Design review of the part built by this model. Coordinates are the model's own, in mm. A direction names the side the tool comes from. Coordinates: 2 decimals unless noted, no trailing zeros. Loops run counter-clockwise (first coordinate to the right, second up) from the corner with the lowest first, then second, coordinate; pieces in that order, holes last. Notation, with made-up numbers: (86, 33.5) -> (132, 33.5) arc R17 ccw to (132, 52.5) -> close; hole circle Ø3 at (-21, 51.25). An arc over 180 degrees is marked (long way). Use CSV: the item, a comma, the result in double quotes.
Autodesk Inventor part; units mm, degrees
ref_plane "YZ Plane" through (0, 0, 0) normal (1, 0, 0) x (0, 1, 0)
ref_plane "XZ Plane" through (0, 0, 0) normal (0, 1, 0) x (-1, 0, 0)
ref_plane "XY Plane" through (0, 0, 0) normal (0, 0, 1) x (1, 0, 0)
sketch "Sketch1" plane through (0, 0, 0) normal (0, 0, 1) x (1, 0, 0)
  circle A0 centre (482.6, 12.7) radius 3.302
  circle A1 centre (508, 241.3) radius 3.302
  circle A2 centre (482.6, 241.3) radius 3.302
  circle A3 centre (355.6, 241.3) radius 3.302
  circle A4 centre (330.2, 241.3) radius 3.302
  circle A5 centre (127, 63.5) radius 3.175
  circle A6 centre (127, 241.3) radius 3.175
  line L0 (427.3692, 9.8745) -> (431.8594, 5.3844)
  line L1 (431.8594, 5.3844) -> (485.7409, 59.2659)
  line L2 (485.7409, 59.2659) -> (481.2508, 63.7561)
  circle A7 centre (330.2, 63.5) radius 3.302
  circle A8 centre (254, 241.3) radius 3.302
  circle A9 centre (279.4, 63.5) radius 3.302
  circle A10 centre (355.6, 63.5) radius 3.302
  circle A11 centre (508, 63.5) radius 3.302
  circle A12 centre (355.6, 12.7) radius 3.302
  circle A13 centre (508, 12.7) radius 3.302
  line L3 (0, 254) -> (76.2, 254)
  line L4 (76.2, 254) -> (76.2, 260.35)
  line L5 (76.2, 260.35) -> (152.4, 260.35)
  line L6 (152.4, 260.35) -> (152.4, 254)
  line L7 (152.4, 254) -> (228.6, 254)
  line L8 (228.6, 254) -> (228.6, 260.35)
  line L9 (228.6, 260.35) -> (520.7, 260.35)
  line L10 (520.7, 260.35) -> (520.7, 0)
  line L11 (520.7, 0) -> (342.9, 0)
  line L12 (228.6, 44.45) -> (228.6, 50.8)
  line L13 (228.6, 50.8) -> (152.4, 50.8)
  line L14 (152.4, 50.8) -> (152.4, 44.45)
  line L15 (152.4, 44.45) -> (76.2, 44.45)
  line L16 (76.2, 44.45) -> (76.2, 50.8)
  line L17 (76.2, 50.8) -> (0, 50.8)
  line L18 (0, 50.8) -> (0, 254)
  line L19 (490.8349, 111.3178) -> (383.0718, 219.0809)
  line L20 (383.0718, 219.0809) -> (387.562, 223.571)
  line L21 (387.562, 223.571) -> (495.3, 115.7829)
  line L22 (495.3, 115.7829) -> (490.8349, 111.3178)
  line L23 (427.3692, 9.8745) -> (481.2508, 63.7561)
  circle A14 centre (279.4, 241.3) radius 3.302
  circle A15 centre (381, 241.3) radius 3.302
  circle A16 centre (254, 63.5) radius 3.302
  circle A17 centre (304.8, 241.3) radius 3.302
  circle A18 centre (304.8, 63.5) radius 3.302
  line L24 (266.7, 0) -> (342.9, 0)
  line L25 (266.7, 0) -> (266.7, 44.45)
  line L26 (228.6, 44.45) -> (266.7, 44.45)
  circle A19 centre (279.4, 12.7) radius 3.302
  point P0 (0, 0)
extrude "Extrusion2" add sketch "Sketch1" along normal blind 6.35
properties part number "vrRig_v8_side"
Item 1: To check wall thickness, follow line 1 along Y through (x, z) = (127, 2.75) (3 decimals); line 2 along Y through (x, z) = (304.8, 4); line 3 along Y through (x, z) = (508, 2.5). State the ranges of each line that lie inside material, in increasing order.
Checked values:
line 1,"44.45 to 60.325, 66.675 to 238.125, 244.475 to 260.35"
line 2,"0 to 60.2, 66.8 to 238, 244.6 to 260.35"
line 3,"0 to 9.4, 16 to 60.2, 66.8 to 238, 244.6 to 260.35"
Item 2: Add section B-B (x = 408). Give the boundary of the cut face in (y, z).
Checked values:
outline,"(0, 0) -> (194.15, 0) -> (194.15, 6.35) -> (0, 6.35) -> close; (203.12, 0) -> (260.35, 0) -> (260.35, 6.35) -> (203.12, 6.35) -> close"
Item 3: Add section C-C (z = 5). State how many separate pieces and enclosed holes the cut face has, then the cut area to 3 significant figures.
Checked values:
separate pieces,"1"
enclosed holes,"22"
area,"120,000 mm^2"
Item 4: Draft analysis for pull direction X (two halves, no side actions). For faces 1 (the face through (440.68, 170.43, 3.13)), 2 (the face through (437.708, 164.445, 3.131)), 3 (the face through (257, 132, 0)), state which applies: pulls with the +X half, pulls with the -X half, needs draft (parallel to the pull), parting line crosses it, or undercut.
Checked values:
face 1,"undercut"
face 2,"undercut"
face 3,"needs draft"
Item 5: Add section D-D (x = 464). Give the boundary of the cut face in (y, z) (3 decimals), then the cut area to 3 significant figures.
Checked values:
outline,"(0, 0) -> (37.525, 0) -> (37.525, 6.35) -> (0, 6.35) -> close; (46.505, 0) -> (138.153, 0) -> (138.153, 6.35) -> (46.505, 6.35) -> close; (147.097, 0) -> (260.35, 0) -> (260.35, 6.35) -> (147.097, 6.35) -> close"
area,"1,540 mm^2"
Item 6: Machinability: for faces 4 (the face through (257, 132, 6.35)), 5 (the face through (458.423, 31.948, 3.131)), which of the approach directions +Z, -Z, +X, -X, +Y, -Y give a long, thin tool a straight path to every point of the face, cutting with its end or side? Answer none if there is none.
Checked values:
face 4,"+Z, +X, -X, +Y, -Y"
face 5,"+Z, -Z"
Item 7: Clearance check with flat-ended pins moving along their axes: pin 1 (4 mm diameter, centred on x = 52.5, y = 209, fed in from -Z); pin 2 (1.9 mm diameter, centred on x = 180.5, z = 3.5, fed in from +Y); pin 3 (1.9 mm diameter, centred on x = 49.5, z = 4, fed in from -Y); pin 4 (1.9 mm diameter, centred on y = 48.5, z = 2.5, fed in from -X). State where each tip first meets the part, or that it passes through.
Checked values:
pin 1,"z = 0"
pin 2,"y = 254"
pin 3,"y = 50.8"
pin 4,"x = 76.2"
Item 8: Add section A-A (y = 28). Give the boundary of the cut face in (x, z) (3 decimals), then the cut area to 3 significant figures.
Checked values:
outline,"(266.7, 0) -> (445.495, 0) -> (445.495, 6.35) -> (266.7, 6.35) -> close; (454.475, 0) -> (520.7, 0) -> (520.7, 6.35) -> (454.475, 6.35) -> close"
area,"1,560 mm^2"
